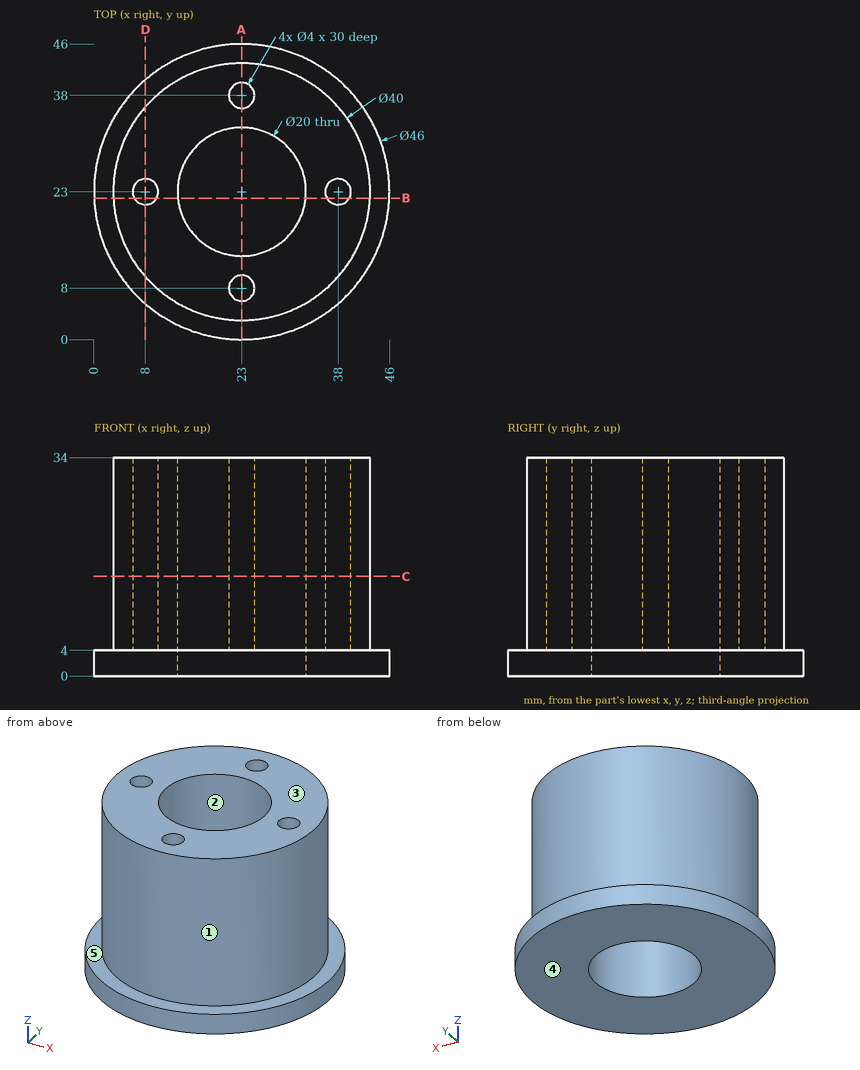
Job drawing, mm, ordinate dimensions from the low corner. One solid piece. A direction names the side the tool comes from. Round coordinates to 2 decimals unless told otherwise and drop trailing zeros. Write each loop counter-clockwise with the first axis right and the second up, starting at its lowest first coordinate (ties: lowest second). Pieces come first, ordered by that corner, then holes. Notation, with made-up numbers: (3, 62) -> (23, 62) arc R5 cw to (23, 71) -> close; hole circle Ø11 at (51.25, -8.75). An arc over 180 degrees is marked (long way). Answer as CSV lines item,"result".
1. Slice it at C-C, the plane z = 15.5. List the corners of the cut face in (x, y).
Resolved:
outline,"circle Ø40 at (23, 23); hole circle Ø4 at (8, 23); hole circle Ø20 at (23, 23); hole circle Ø4 at (23, 8); hole circle Ø4 at (23, 38); hole circle Ø4 at (38, 23)"
2. Slice it at B-B, the plane y = 22. List the corners of the cut face in (x, z).
Resolved:
outline,"(0.02, 0) -> (13.05, 0) -> (13.05, 34) -> (9.73, 34) -> (9.73, 4) -> (6.27, 4) -> (6.27, 34) -> (3.03, 34) -> (3.03, 4) -> (0.02, 4) -> close; (32.95, 0) -> (45.98, 0) -> (45.98, 4) -> (42.97, 4) -> (42.97, 34) -> (39.73, 34) -> (39.73, 4) -> (36.27, 4) -> (36.27, 34) -> (32.95, 34) -> close"
3. Slice it at A-A, the plane x = 23. List the corners of the cut face in (y, z).
Resolved:
outline,"(0, 0) -> (13, 0) -> (13, 34) -> (10, 34) -> (10, 4) -> (6, 4) -> (6, 34) -> (3, 34) -> (3, 4) -> (0, 4) -> close; (33, 0) -> (46, 0) -> (46, 4) -> (43, 4) -> (43, 34) -> (40, 34) -> (40, 4) -> (36, 4) -> (36, 34) -> (33, 34) -> close"
4. Mould opens along X. For the marked faces 1, 2 and 3 say: +X half, -X half, draft (parallel to the pull), parting line (faces both ways), or undercut.
Resolved:
face 1,"parting line"
face 2,"undercut"
face 3,"draft"
5. Pin check, flat tips, straight feed: pin 1 Ø5 at (x, z) = (12, 18.5) entering from +Y; pin 2 Ø1 at (x, z) = (19, 10.5) entering from +Y; pin 3 Ø3 at (x, y) = (41, 41) entering from +Z; pin 4 Ø6 at (y, z) = (5.5, 26) entering from -X (3 decimals). Stop position of each tip, or through.
Resolved:
pin 1,"y = 41.1"
pin 2,"y = 42.69"
pin 3,"through"
pin 4,"x = 9.225"
6. Drill centre lines: line 1 (Y direction, x = 23, z = 9.5); line 2 (Y direction, x = 24.5, z = 23); line 3 (Y direction, x = 38, z = 15.5). Where is each one in solid material? Low to high.
Resolved:
line 1,"3 to 6, 10 to 13, 33 to 36, 40 to 43"
line 2,"3.06 to 6.68, 9.32 to 13.11, 32.89 to 36.68, 39.32 to 42.94"
line 3,"9.77 to 21, 25 to 36.23"
7. Slice it at D-D, the plane x = 8. List the corners of the cut face in (y, z).
Resolved:
outline,"(5.56, 0) -> (40.44, 0) -> (40.44, 4) -> (36.23, 4) -> (36.23, 34) -> (25, 34) -> (25, 4) -> (21, 4) -> (21, 34) -> (9.77, 34) -> (9.77, 4) -> (5.56, 4) -> close"
8. Tool access for the marked faces 4 and 5: list every direction of +Z, -Z, +X, -X, +Y, -Y with a clear straight run to the whole face (end or side of a thin tool).
Resolved:
face 4,"-Z, +X, -X, +Y, -Y"
face 5,"+Z"
